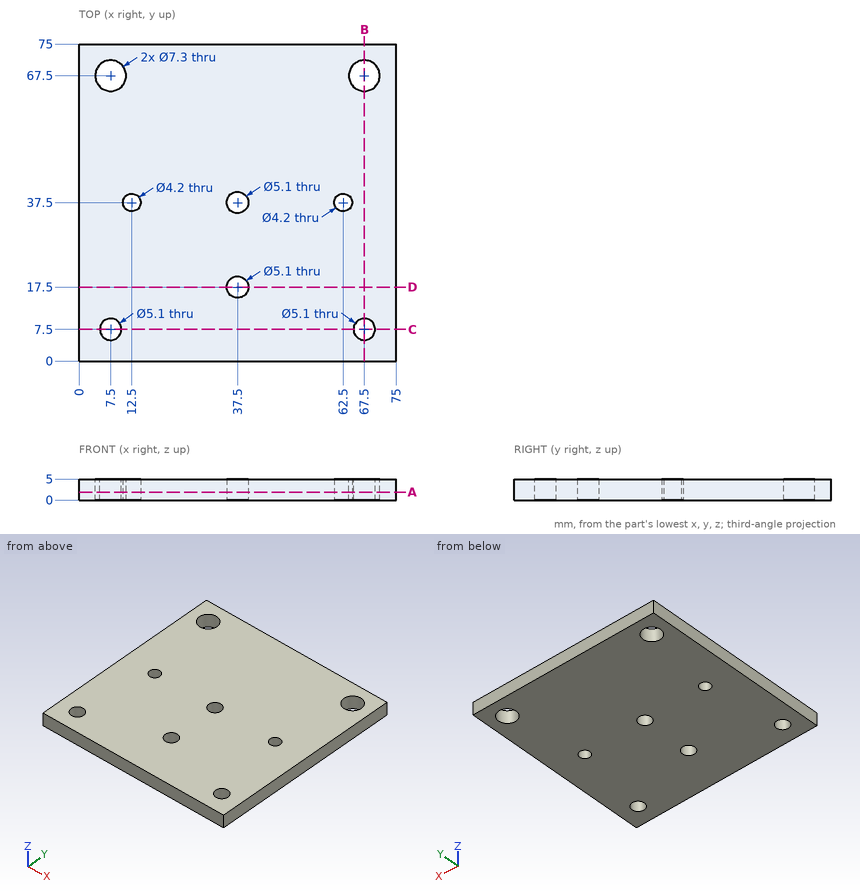
Geometry: see drawing. Coordinates: mm, zero at the bounding-box minimum. Give positions to 0.01 mm unless a question says otherwise; leave off trailing zeros. Loops run counter-clockwise (first coordinate to the right, second up) from the corner with the lowest first, then second, coordinate; pieces in that order, holes last. Notation, with made-up numbers: (86, 26) - (138, 26) arc R18 ccw to (138, 32) - close; hole circle Ø5 at (5, 0). An arc over 180 degrees is marked (long way). Answer as CSV lines item,"result". Start each with the question number.
1. Section C-C, the plane y = 7.5. Return loops of the section in (x, z).
2. Section D-D, the plane y = 17.5. Return loops of the section in (x, z).
3. Section B-B, the plane x = 67.5. Return loops of the section in (y, z).
4. Ray query, L1, parallel to X at y = 67.5, z = 2.25; L2, parallel to Y at x = 37.5, z = 2.6; L3, parallel to X at y = 7.5, z = 3.8. Return the intervals inside material, ascending.
5. Pin query (flat end, axial travel): P1, Ø8, axis at x = 37.5, y = 17.5, coming from the +Z side; P2, Ø4.5, axis at x = 7.5, y = 7.5, coming from the +Z side. Return the tip coordinate at first contact, or that it passes through.
6. Section A-A, the plane z = 1.9. Give the number of separate pieces and of enclosed holes in the cut face, plus the area to 3 significant figures.
Answers:
1,outline,"(0, 0) - (4.95, 0) - (4.95, 5) - (0, 5) - close; (10.05, 0) - (64.95, 0) - (64.95, 5) - (10.05, 5) - close; (70.05, 0) - (75, 0) - (75, 5) - (70.05, 5) - close"
2,outline,"(0, 0) - (34.95, 0) - (34.95, 5) - (0, 5) - close; (40.05, 0) - (75, 0) - (75, 5) - (40.05, 5) - close"
3,outline,"(0, 0) - (4.95, 0) - (4.95, 5) - (0, 5) - close; (10.05, 0) - (63.85, 0) - (63.85, 5) - (10.05, 5) - close; (71.15, 0) - (75, 0) - (75, 5) - (71.15, 5) - close"
4,L1,"x = 0 to 3.85, 11.15 to 63.85, 71.15 to 75"
4,L2,"y = 0 to 14.95, 20.05 to 34.95, 40.05 to 75"
4,L3,"x = 0 to 4.95, 10.05 to 64.95, 70.05 to 75"
5,P1,"stops at z = 5"
5,P2,"passes through"
6,separate pieces,"1"
6,enclosed holes,"8"
6,area,"5,430 mm2"
